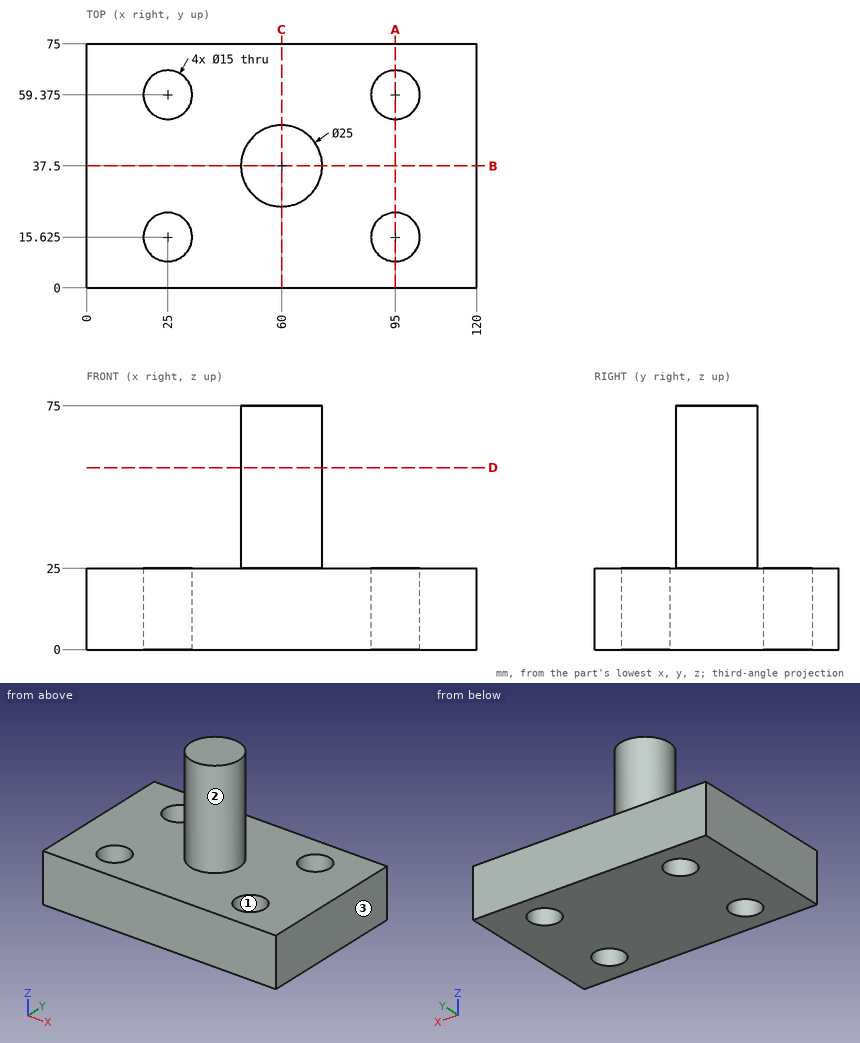
Input: dimensioned drawing with shaded views. Units: mm. Origin: part minimum x, y, z. Give positions to 0.01 mm unless a question says otherwise; leave off trailing zeros. Order: outer loops, then holes, each group sorted by start corner. A loop starts at its lowest first (then second) coordinate and runs counter-clockwise, first axis right, second up. Notation, with made-up numbers: (70.5, 72) -> (124.5, 72) arc R17 cw to (124.5, 84) -> close; hole circle Ø2 at (-25.75, -8.5). An arc over 180 degrees is marked (long way). Write item = value, one per line.
Item 1: Mould query, pull axis Y, two halves, no side actions, for the marked faces 1, 2 and 3. Classes: +Y half, -Y half, draft (parallel to the pull), parting line (faces both ways), or undercut.
Check result:
face_1 = undercut
face_2 = parting line
face_3 = draft
Item 2: Section query D-D (z = 56). Output: boundary loops of the cut face in (x, y).
Check result:
outline = circle Ø25 at (60, 37.5)
Item 3: Section query A-A (x = 95). Output: boundary loops of the cut face in (y, z) (3 decimals).
Check result:
outline = (0, 0) -> (8.125, 0) -> (8.125, 25) -> (0, 25) -> close; (23.125, 0) -> (51.875, 0) -> (51.875, 25) -> (23.125, 25) -> close; (66.875, 0) -> (75, 0) -> (75, 25) -> (66.875, 25) -> close
Item 4: Ray query, probe 1 along X at (y, z) = (16, 4.5); probe 2 along Y at (x, z) = (95, 6) (3 decimals); probe 3 along X at (y, z) = (19, 12.5). Return the intervals inside material, ascending.
Check result:
probe_1 = 0 to 17.51, 32.49 to 87.51, 102.49 to 120
probe_2 = 0 to 8.125, 23.125 to 51.875, 66.875 to 75
probe_3 = 0 to 18.3, 31.7 to 88.3, 101.7 to 120
Item 5: Section query C-C (x = 60). Output: boundary loops of the cut face in (y, z), then the cut area to 4 significant figures.
Check result:
outline = (0, 0) -> (75, 0) -> (75, 25) -> (50, 25) -> (50, 75) -> (25, 75) -> (25, 25) -> (0, 25) -> close
area = 3,125 mm²
Item 6: Section query B-B (y = 37.5). Output: boundary loops of the cut face in (x, z), then the cut area to 3 significant figures.
Check result:
outline = (0, 0) -> (120, 0) -> (120, 25) -> (72.5, 25) -> (72.5, 75) -> (47.5, 75) -> (47.5, 25) -> (0, 25) -> close
area = 4,250 mm²
